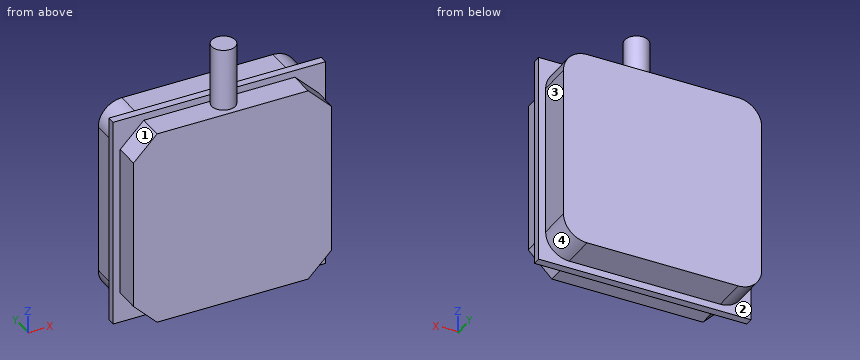
```python
from build123d import *

# Parameters (mm, degrees)
SKETCH1_W           = 27
SKETCH1_H           = 27
BOSS_EXTRUDE1_DEPTH = 1
BOSS_EXTRUDE2_DEPTH = 4.3
BOSS_EXTRUDE3_DEPTH = 3.2
SKETCH4_R           = 1.5
BOSS_EXTRUDE5_DEPTH = 8


with BuildPart() as part:
    # Sketch1 → Boss-Extrude1 (new body)
    with BuildSketch(Plane(origin=(0, 0, 0), x_dir=(1, 0, 0), z_dir=(0, 1, 0))):
        with Locations((13.5, 13.5)):
            Rectangle(SKETCH1_W, SKETCH1_H)
    extrude(amount=BOSS_EXTRUDE1_DEPTH)

    # Sketch2 → Boss-Extrude2 (add)
    with BuildSketch(Plane(origin=(0, 1, 0), x_dir=(1, 0, 0), z_dir=(0, 1, 0))):
        with BuildLine():
            Line((3.9, 26.1), (23.1, 26.1))
            ThreePointArc((23.1, 26.1), (25.221320344, 25.221320344), (26.1, 23.1))
            Line((26.1, 23.1), (26.1, 3.9))
            ThreePointArc((26.1, 3.9), (25.221320344, 1.778679656), (23.1, 0.9))
            Line((23.1, 0.9), (3.9, 0.9))
            ThreePointArc((3.9, 0.9), (1.778679656, 1.778679656), (0.9, 3.9))
            Line((0.9, 3.9), (0.9, 23.1))
            ThreePointArc((0.9, 23.1), (1.778679656, 25.221320344), (3.9, 26.1))
        make_face()
    extrude(amount=BOSS_EXTRUDE2_DEPTH)

    # Sketch3 → Boss-Extrude3 (add)
    with BuildSketch(Plane.XZ):
        Polygon((3.9, -0.9), (23.1, -0.9), (26.1, -3.9), (26.1, -23.1), (23.1, -26.1), (3.9, -26.1), (0.9, -23.1), (0.9, -3.9), align=None)
    extrude(amount=BOSS_EXTRUDE3_DEPTH)

    # Sketch4 → Boss-Extrude5 (add)
    with BuildSketch(Plane.XY.offset(-0.9)):
        with Locations((13.5, -1)):
            Circle(SKETCH4_R)
    extrude(amount=BOSS_EXTRUDE5_DEPTH)


solid = part.part
```
Model file for the job. Use its own axes, mm. Face numbers are marked on the shaded views. A direction names the side the tool comes from. Give positions to 0.01 mm unless a question says otherwise; leave off trailing zeros. Loops run counter-clockwise (first coordinate to the right, second up) from the corner with the lowest first, then second, coordinate; pieces in that order, holes last. Notation, with made-up numbers: (34, 86.25) - (66, 86.25) arc R17 cw to (66, 102.25) - close; hole circle Ø11 at (32, 34.5). An arc over 180 degrees is marked (long way). One line per item, written item: value. Start each with the question number.
1. Slice it at A-A (x = 13.5). List the corners of the cut face in (y, z).
2. Probe L1, parallel to X at y = -1.5, z = -21; L2, parallel to Z at x = 20, y = 1.75; L3, parallel to Z at x = 14.25, y = -1.5. List the from-to ranges inside material, lowest first. Write a range as from..to.
3. Pin check, flat tips, straight feed: pin 1 (4.5 mm diameter, centred on x = 16, y = 2, fed in from +Z); pin 2 (1 mm diameter, centred on y = -1.5, z = -13, fed in from +X); pin 3 (1.6 mm diameter, centred on x = 11.5, y = -1.5, fed in from -Z). Stop position of each tip, or through.
4. Slice it at B-B (y = 4.75). List the corners of the cut face in (x, z).
5. Which spindle directions (+Z, -Z, +X, -X, +Y, -Y) get a long thin tool onto all of the face, cutting with end or side? Do the marked faces 1, 2, 3 and 4. Say none if no direction does.
6. Slice it at D-D (y = -1). List the corners of the cut face in (x, z).
7. Slice it at C-C (z = -14). List the corners of the cut face in (x, y).
Solution:
1. outline: (-3.2, -26.1) - (0, -26.1) - (0, -27) - (1, -27) - (1, -26.1) - (5.3, -26.1) - (5.3, -0.9) - (1, -0.9) - (1, 0) - (0.5, 0) - (0.5, 7.1) - (-2.5, 7.1) - (-2.5, -0.9) - (-3.2, -0.9) - close
2. L1: x = 0.9..26.1
2. L2: z = -26.1..-0.9
2. L3: z = -26.1..7.1
3. pin 1: stops at z = 0
3. pin 2: stops at x = 26.1
3. pin 3: stops at z = -26.1
4. outline: (0.9, -23.1) arc R3 ccw to (3.9, -26.1) - (23.1, -26.1) arc R3 ccw to (26.1, -23.1) - (26.1, -3.9) arc R3 ccw to (23.1, -0.9) - (3.9, -0.9) arc R3 ccw to (0.9, -3.9) - close
5. face 1: +Z, -X, -Y
5. face 2: +Y
5. face 3: +Z, -Z, +X, +Y
5. face 4: -Z, +X, +Y
6. outline: (0.9, -23.1) - (3.9, -26.1) - (23.1, -26.1) - (26.1, -23.1) - (26.1, -3.9) - (23.1, -0.9) - (15, -0.9) - (15, 7.1) - (12, 7.1) - (12, -0.9) - (3.9, -0.9) - (0.9, -3.9) - close
7. outline: (0, 0) - (0.9, 0) - (0.9, -3.2) - (26.1, -3.2) - (26.1, 0) - (27, 0) - (27, 1) - (26.1, 1) - (26.1, 5.3) - (0.9, 5.3) - (0.9, 1) - (0, 1) - close
